Design review of the part shown in the three views and the two pictorial views. Dimensions are in mm from the part's minimum x, y and z. A direction names the side the tool comes from. Round coordinates to 2 decimals unless told otherwise and drop trailing zeros. Order: outer loops, then holes, each group sorted by start corner. A loop starts at its lowest first (then second) coordinate and runs counter-clockwise, first axis right, second up. Notation, with made-up numbers: (-30.75, 67) - (15.25, 67) arc R20 ccw to (15.25, 88) - close; hole circle Ø10 at (59.25, 7). An arc over 180 degrees is marked (long way). One line per item, written item: value.
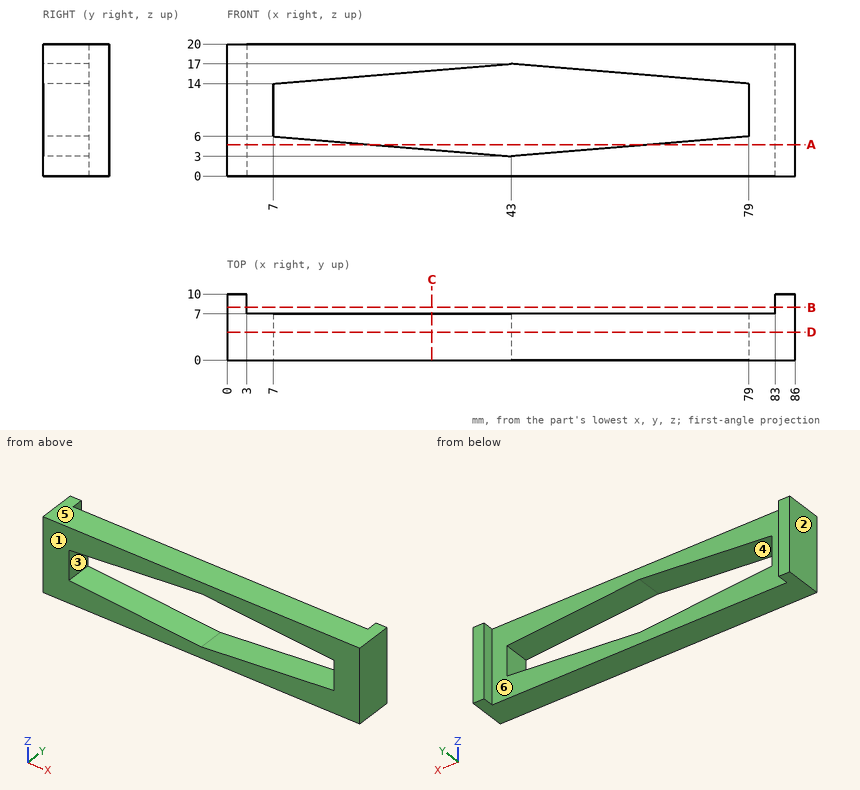
Item 1: For P1, Ø10, axis at x = 54.5, z = 11.5, coming from the +Y side, flat-tipped, find the tip position at first contact; note if it passes through.
Returned:
P1: y = 7
Item 2: The part is to be moulded in two halves that separate along X. For the marked faces 1, 2 and 3, say which applies: +X half, -X half, draft (parallel to the pull), parting line (faces both ways), or undercut.
Returned:
face 1: draft
face 2: -X half
face 3: undercut
Item 3: Take a section at D-D (y = 4.25). Write out the cut boundary in (x, z).
Returned:
outline: (0, 0) - (86, 0) - (86, 20) - (0, 20) - close; hole (7, 6) - (43, 3) - (79, 6) - (79, 14) - (43, 17) - (7, 14) - close
Item 4: Take a section at A-A (z = 4.75). Write out the cut boundary in (x, y), plus the area to 3 significant figures.
Returned:
outline: (0, 0) - (22, 0) - (22, 7) - (3, 7) - (3, 10) - (0, 10) - close; (64, 0) - (86, 0) - (86, 10) - (83, 10) - (83, 7) - (64, 7) - close
area: 326 mm^2
Item 5: Wall thickness on line 1 (X direction, y = 6.5, z = 6.5); line 2 (X direction, y = 9, z = 3.75); line 3 (Y direction, x = 26, z = 2): over which ranges is each line inside the solid? List them lowest first.
Returned:
line 1: 0 to 7, 79 to 86
line 2: 0 to 3, 83 to 86
line 3: 0 to 7
Item 6: Take a section at B-B (y = 8). Write out the cut boundary in (x, z).
Returned:
outline: (0, 0) - (3, 0) - (3, 20) - (0, 20) - close; (83, 0) - (86, 0) - (86, 20) - (83, 20) - close
Item 7: Machinability: for the marked faces 4, 5 and 6, which of the approach directions +Z, -Z, +X, -X, +Y, -Y give a long, thin tool a straight path to every point of the face, cutting with its end or side? Answer none if there is none.
Returned:
face 4: +Y, -Y
face 5: +Z, +X, -X, +Y, -Y
face 6: +Z, -Z, +Y
Item 8: Take a section at C-C (x = 31). Write out the cut boundary in (y, z).
Returned:
outline: (0, 0) - (7, 0) - (7, 4) - (0, 4) - close; (0, 16) - (7, 16) - (7, 20) - (0, 20) - close
